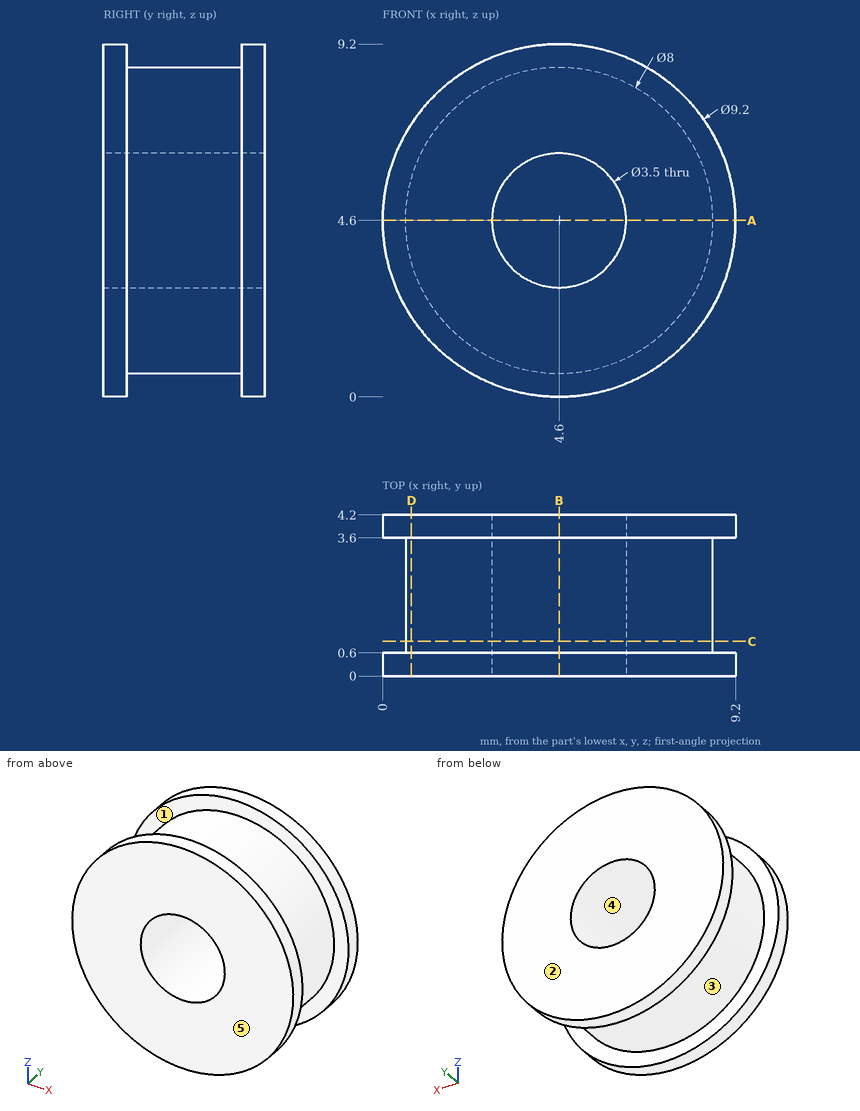
Verification items for this drawing (mm, ordinates from the low corner). A direction names the side the tool comes from. Round coordinates to 2 decimals unless told otherwise and drop trailing zeros. Order: outer loops, then holes, each group sorted by start corner. A loop starts at its lowest first (then second) coordinate and runs counter-clockwise, first axis right, second up. Notation, with made-up numbers: (19, 29) - (49, 29) arc R23 ccw to (49, 58) - close; hole circle Ø8 at (71.25, -30). An arc over 180 degrees is marked (long way). Use CSV: the item, a comma, the result in double quotes. Start each with the question number.
1) Access from +Z, -Z, +X, -X, +Y, -Y to the whole of each face (thin tool, end or side, straight path). Record for the marked faces 1 and 2.
2) Section check B-B, the plane x = 4.6. Record the cut outline in (y, z), plus the area to 3 significant figures.
3) Section check D-D, the plane x = 0.75. Record the cut outline in (y, z).
4) Section check C-C, the plane y = 0.9. Record the cut outline in (x, z).
5) Go/stop test with flat-tipped pins: P1, Ø1, axis at x = 7.5, y = 1, coming from the -Z side; P2, Ø2, axis at x = 3.5, y = 1, coming from the +Z side; P3, Ø1, axis at x = 7.5, y = 1.5, coming from the -Z side. Record where each tip stops, or that it passes through.
6) Section check A-A, the plane z = 4.6. Record the cut outline in (x, y).
7) Mould release check, pull along Z, two halves, no side actions. Record for the marked faces 3, 4 and 5: +Z half, -Z half, draft (parallel to the pull), parting line (faces both ways), or undercut.
8) Thickness scan on L1, parallel to X at y = 2.5, z = 4.6; L2, parallel to Y at x = 7.5, z = 7.5; L3, parallel to Z at x = 3, y = 0.4. Record the ranges inside material, lowest first.
Answers:
1,face 1,"none"
1,face 2,"+Z, -Z, +X, -X, +Y"
2,outline,"(0, 0) - (0.6, 0) - (0.6, 0.6) - (3.6, 0.6) - (3.6, 0) - (4.2, 0) - (4.2, 2.85) - (0, 2.85) - close; (0, 6.35) - (4.2, 6.35) - (4.2, 9.2) - (3.6, 9.2) - (3.6, 8.6) - (0.6, 8.6) - (0.6, 9.2) - (0, 9.2) - close"
2,area,"20.3 mm²"
3,outline,"(0, 2.08) - (0.6, 2.08) - (0.6, 3.51) - (3.6, 3.51) - (3.6, 2.08) - (4.2, 2.08) - (4.2, 7.12) - (3.6, 7.12) - (3.6, 5.69) - (0.6, 5.69) - (0.6, 7.12) - (0, 7.12) - close"
4,outline,"circle Ø8 at (4.6, 4.6); hole circle Ø3.5 at (4.6, 4.6)"
5,P1,"stops at z = 0.81"
5,P2,"stops at z = 9.2"
5,P3,"stops at z = 1.4"
6,outline,"(0, 0) - (2.85, 0) - (2.85, 4.2) - (0, 4.2) - (0, 3.6) - (0.6, 3.6) - (0.6, 0.6) - (0, 0.6) - close; (6.35, 0) - (9.2, 0) - (9.2, 0.6) - (8.6, 0.6) - (8.6, 3.6) - (9.2, 3.6) - (9.2, 4.2) - (6.35, 4.2) - close"
7,face 3,"parting line"
7,face 4,"undercut"
7,face 5,"draft"
8,L1,"x = 0.6 to 2.85, 6.35 to 8.6"
8,L2,"y = 0 to 0.6, 3.6 to 4.2"
8,L3,"z = 0.29 to 3.89, 5.31 to 8.91"
